from build123d import *

# Parameters (mm, degrees)
EXTRUDE_1_DEPTH     = 170
SKETCH_2_R          = 60
CUT_EXTRUDE_1_DEPTH = 180
SKETCH_3_R          = 30
CUT_EXTRUDE_2_DEPTH = 180


with BuildPart() as part:
    # 草图1 → 凸台-拉伸1 (new body)
    with BuildSketch(Plane.XY):
        Polygon((-180, 0), (0, 0), (0, -150), (8, -150), (8, 8), (-180, 8), align=None)
    extrude(amount=EXTRUDE_1_DEPTH)

    # 草图2 → 切除-拉伸1 (cut)
    with BuildSketch(Plane(origin=(0, 8, 0), x_dir=(1, 0, 0), z_dir=(0, 1, 0))):
        with Locations(Location((-90, -85, 0), (0, 0, 180))):
            Circle(SKETCH_2_R)
        with BuildLine():
            ThreePointArc((-90, -170), (-175, -85), (-90, 0))
            Line((-90, 0), (-180, 0))
            Line((-180, 0), (-180, -170))
            Line((-180, -170), (-90, -170))
        make_face()
    extrude(amount=-CUT_EXTRUDE_1_DEPTH, mode=Mode.SUBTRACT)

    # 草图3 → 切除-拉伸2 (cut)
    with BuildSketch(Plane(origin=(8, 0, 0), x_dir=(0, 0, -1), z_dir=(1, 0, 0))):
        with Locations(Location((-85, -70, 0), (0, 0, 90))):
            Circle(SKETCH_3_R)
    extrude(amount=-CUT_EXTRUDE_2_DEPTH, mode=Mode.SUBTRACT)


solid = part.part
For this review, take the finished solid that the model builds, in its own axes (mm). Round coordinates to 2 decimals unless told otherwise and drop trailing zeros. Write each loop counter-clockwise with the first axis right and the second up, starting at its lowest first coordinate (ties: lowest second). Pieces come first, ordered by that corner, then holes. Notation, with made-up numbers: (-18, 20.5) -> (6, 20.5) arc R19 cw to (6, 40.5) -> close; hole circle Ø2 at (23, 44). An arc over 180 degrees is marked (long way). Use CSV: the item, a comma, the result in double quotes.
(1) Consider section A-A, the plane y = -70. Give the boundary of the cut face in (x, z), plus the area to 3 significant figures.
Computed values:
outline,"(0, 0) -> (8, 0) -> (8, 55) -> (0, 55) -> close; (0, 115) -> (8, 115) -> (8, 170) -> (0, 170) -> close"
area,"880 mm²"
(2) Draft analysis for pull direction X (two halves, no side actions). For faces 1 (the face through (8, -37, 84)), 2 (the face through (-76.993, 4.056, 26.427)), 3 (the face through (-30, 0, 65)), 4 (the face through (0, -107, 84)), state which applies: +X half, -X half, draft (parallel to the pull), parting line (faces both ways), or undercut.
Computed values:
face 1,"+X half"
face 2,"undercut"
face 3,"draft"
face 4,"-X half"
(3) To check wall thickness, follow L1, parallel to Z at x = -90, y = 5.5; L2, parallel to Z at x = 4.25, y = -70; L3, parallel to X at y = -39, z = 152. State the ranges of each line that lie inside material, in increasing order. Write a range as [from, to].
Computed values:
L1,"[0, 25], [145, 170]"
L2,"[0, 55], [115, 170]"
L3,"[0, 8]"
(4) Consider section D-D, the plane z = 133.5. Give the boundary of the cut face in (x, y), plus the area to 3 significant figures.
Computed values:
outline,"(-159.81, 0) -> (-125.32, 0) -> (-125.32, 8) -> (-159.81, 8) -> close; (-54.68, 0) -> (0, 0) -> (0, -150) -> (8, -150) -> (8, 8) -> (-54.68, 8) -> close"
area,"1,980 mm²"
(5) Consider section C-C, the plane x = -124.5. Give the boundary of the cut face in (y, z).
Computed values:
outline,"(0, 7.32) -> (8, 7.32) -> (8, 35.91) -> (0, 35.91) -> close; (0, 134.09) -> (8, 134.09) -> (8, 162.68) -> (0, 162.68) -> close"
(6) Consider section B-B, the plane z = 85. Give the boundary of the cut face in (x, y), plus the area to 3 significant figures.
Computed values:
outline,"(-175, 0) -> (-150, 0) -> (-150, 8) -> (-175, 8) -> close; (-30, 0) -> (0, 0) -> (0, -40) -> (8, -40) -> (8, 8) -> (-30, 8) -> close; (0, -150) -> (8, -150) -> (8, -100) -> (0, -100) -> close"
area,"1,220 mm²"
